Geometry: final body of the model. Coordinates: model frame, mm. A direction names the side the tool comes from. Give positions to 0.01 mm unless a question says otherwise; leave off trailing zeros. Write each loop counter-clockwise with the first axis right and the second up, starting at its lowest first coordinate (ties: lowest second). Pieces come first, ordered by that corner, then holes.
```python
from build123d import *

# Parameters (mm, degrees)
CROQUIS1_R              = 8
CROQUIS1_R_2            = 4
CROQUIS1_R_3            = 2.5
CROQUIS1_R_4            = 1.75
SALIENTE_EXTRUIR1_DEPTH = 5


with BuildPart() as part:
    # Croquis1 → Saliente-Extruir1 (new body)
    with BuildSketch(Plane(origin=(0, 0, 0), x_dir=(0, 0, -1), z_dir=(1, 0, 0))):
        Polygon((150, 150), (0, 50), (0, 0), (50, 0), (50, -10), (150, -10), (150, 0), (200, 0), (200, 150), (192.5, 150), (192.5, 155), (157.5, 155), (157.5, 150), align=None)
        with Locations((175, 125)):
            Circle(CROQUIS1_R, mode=Mode.SUBTRACT)
        with Locations((175, 20)):
            Circle(CROQUIS1_R_2, mode=Mode.SUBTRACT)
        with Locations((150, 35)):
            Circle(CROQUIS1_R_2, mode=Mode.SUBTRACT)
        with Locations((175, 143.25)):
            Circle(CROQUIS1_R_3, mode=Mode.SUBTRACT)
        with Locations((175, 106.75)):
            Circle(CROQUIS1_R_3, mode=Mode.SUBTRACT)
        with Locations((100, 35)):
            Circle(CROQUIS1_R, mode=Mode.SUBTRACT)
        with Locations((84.5, 60.685599078)):
            Circle(CROQUIS1_R_2, mode=Mode.SUBTRACT)
        with Locations((100, 53.25)):
            Circle(CROQUIS1_R_3, mode=Mode.SUBTRACT)
        with Locations((100, 16.75)):
            Circle(CROQUIS1_R_3, mode=Mode.SUBTRACT)
        with Locations((84.5, 50.5)):
            Circle(CROQUIS1_R_4, mode=Mode.SUBTRACT)
        with Locations((115.5, 50.5)):
            Circle(CROQUIS1_R_4, mode=Mode.SUBTRACT)
        with Locations((115.5, 19.5)):
            Circle(CROQUIS1_R_4, mode=Mode.SUBTRACT)
        with Locations((84.5, 19.5)):
            Circle(CROQUIS1_R_4, mode=Mode.SUBTRACT)
        with Locations((50, 35)):
            Circle(CROQUIS1_R, mode=Mode.SUBTRACT)
        with Locations((50, 53.25)):
            Circle(CROQUIS1_R_3, mode=Mode.SUBTRACT)
        with Locations((50, 16.75)):
            Circle(CROQUIS1_R_3, mode=Mode.SUBTRACT)
        with Locations((34.5, 50.5)):
            Circle(CROQUIS1_R_4, mode=Mode.SUBTRACT)
        with Locations((65.5, 50.5)):
            Circle(CROQUIS1_R_4, mode=Mode.SUBTRACT)
        with Locations((65.5, 19.5)):
            Circle(CROQUIS1_R_4, mode=Mode.SUBTRACT)
        with Locations((34.5, 19.5)):
            Circle(CROQUIS1_R_4, mode=Mode.SUBTRACT)
        Polygon((65, 88.333333333), (139.88452649, 138.256350994), (142.658027472, 134.096099522), (67.773500981, 84.173081862), align=None, mode=Mode.SUBTRACT)
    extrude(amount=SALIENTE_EXTRUIR1_DEPTH)


solid = part.part
```
Item 1: Section B-B, the plane z = -100. Return the cut outline in (x, y).
Found:
outline: (0, -10) - (5, -10) - (5, 14.25) - (0, 14.25) - close; (0, 19.25) - (5, 19.25) - (5, 27) - (0, 27) - close; (0, 43) - (5, 43) - (5, 50.75) - (0, 50.75) - close; (0, 55.75) - (5, 55.75) - (5, 105.66) - (0, 105.66) - close; (0, 111.67) - (5, 111.67) - (5, 116.67) - (0, 116.67) - close
Item 2: Line query: L1, parallel to Y at x = 1.8, z = -175; L2, parallel to Y at x = 4.75, z = -66; L3, parallel to Z at x = 2.15, y = 119. Output: solid intervals per line, ascending.
Found:
L1: y = 0 to 16, 24 to 104.25, 109.25 to 117, 133 to 140.75, 145.75 to 155
L2: y = -10 to 17.82, 21.18 to 48.82, 52.18 to 86.83, 89 to 94
L3: z = -200 to -180.29, -169.71 to -120.01, -111 to -103.5
Item 3: Reachability of faces 1 (the face through (2, 0, -25)), 2 (the face through (2, 153, -157.5)), 3 (the face through (2, 0, -175)), 4 (the face through (2.465, 109.484, -105.74)) from +Z, -Z, +X, -X, +Y, -Y: full face, straight path, thin tool, end or side. Return the list, or none.
Found:
face 1: +Z, +X, -X, -Y
face 2: +Z, +X, -X, +Y
face 3: -Z, +X, -X, -Y
face 4: +X, -X
Item 4: Section C-C, the plane y = 106.75. Return the cut outline in (x, z) (3 decimals).
Found:
outline: (0, -200) - (5, -200) - (5, -177.5) - (0, -177.5) - close; (0, -172.5) - (5, -172.5) - (5, -101.639) - (0, -101.639) - close; (0, -92.625) - (5, -92.625) - (5, -85.125) - (0, -85.125) - close
Item 5: Section A-A, the plane y = 35. Return the cut outline in (x, z).
Found:
outline: (0, -200) - (5, -200) - (5, -154) - (0, -154) - close; (0, -146) - (5, -146) - (5, -108) - (0, -108) - close; (0, -92) - (5, -92) - (5, -58) - (0, -58) - close; (0, -42) - (5, -42) - (5, 0) - (0, 0) - close
Item 6: Section D-D, the plane z = -121. Return the cut outline in (x, y), plus the area to 3 significant figures.
Found:
outline: (0, -10) - (5, -10) - (5, 119.66) - (0, 119.66) - close; (0, 125.67) - (5, 125.67) - (5, 130.67) - (0, 130.67) - close
area: 673 mm2
Item 7: Pin query (flat end, axial travel): pin 1 Ø1 at (x, y) = (1, 135.5) entering from +Z; pin 2 Ø2 at (x, y) = (2, 134) entering from +Z; pin 3 Ø2 at (x, y) = (2.5, 73.5) entering from +Z. Return the tip coordinate at first contact, or that it passes through.
Found:
pin 1: stops at z = -127.5
pin 2: stops at z = -124.5
pin 3: stops at z = -33.75
